Check sheet for the modelled part. Datum: model origin and axes. Units: mm. A direction names the side the tool comes from. Round coordinates to 2 decimals unless told otherwise and drop trailing zeros. Write each loop counter-clockwise with the first axis right and the second up, starting at its lowest first coordinate (ties: lowest second). Pieces come first, ordered by that corner, then holes.
Item 1: Depth check by flat-ended pin: pin 1 (5 mm diameter, centred on x = -133.5, z = -11.5, fed in from -Y); pin 2 (5 mm diameter, centred on x = 62.5, y = -26.5, fed in from -Z); pin 3 (4 mm diameter, centred on y = -3, z = -67, fed in from -X). Enter the tip coordinate at first touch or a pass-through.
Item 2: Material ranges on line 1 along Z through (x, y) = (-70, -9.5); line 2 along Y through (x, z) = (110, -3.5); line 3 along X through (y, z) = (-4, 32.5), recorded low to high.
Item 3: Section check D-D, the plane x = 111. Record the cut outline in (y, z).
Item 4: Section check A-A, the plane z = -79. Record the cut outline in (x, y).
Item 5: Set-up check for faces 1 (the flat face through (102.829, -17, -1)), 2 (the flat face through (-4, -15, -95)), 3 (the flat face through (-107.171, -17, -1)): record each of +Z, -Z, +X, -X, +Y, -Y from which the full face is reachable in a straight line by a thin tool's end or side.
Item 6: Section check C-C, the plane y = -17. Record the cut outline in (x, z), plus the area to 3 significant figures.
Item 7: Section check B-B, the plane x = -93.5. Record the cut outline in (y, z).
from build123d import *

# Parameters (mm, degrees)
F0_W     = 210
F0_H     = 190
F1_DEPTH = 40
F2_W     = 330
F2_H     = 310
F3_DEPTH = 30
F4_SIZE  = 10
F5_SIZE  = 5


with BuildPart() as f1:
    # F0 (on Front) → F1 (new body)
    with BuildSketch(Plane.XZ):
        with Locations((-2.170864, 0)):
            Rectangle(F0_W, F0_H)
    extrude(amount=F1_DEPTH)

    # F2 (on face) → F3 (join)
    with BuildSketch(Plane(origin=(0, 0, 0), x_dir=(-1, 0, 0), z_dir=(0, 1, 0))):
        with Locations((2.170864, 0)):
            Rectangle(F2_W, F2_H)
    extrude(amount=F3_DEPTH)

    # F4
    f4_edges = [f1.edges().sort_by_distance(p)[0] for p in [
        (-2.170864, -40, 95),
        (-2.170864, -40, -95),
    ]]
    chamfer(f4_edges, length=F4_SIZE)

    # F5
    f5_edges = [f1.edges().sort_by_distance(p)[0] for p in [
        (-107.170864, -40, 0),
        (102.829136, -40, 0),
    ]]
    chamfer(f5_edges, length=F5_SIZE)


solid = f1.part
Values found:
1. pin 1: stops at y = 0
1. pin 2: stops at z = -95
1. pin 3: stops at x = -107.17
2. line 1: z = -95 to 95
2. line 2: y = 0 to 30
2. line 3: x = -107.17 to 102.83
3. outline: (0, -155) - (30, -155) - (30, 155) - (0, 155) - close
4. outline: (-167.17, 0) - (-107.17, 0) - (-107.17, -35) - (-102.17, -40) - (97.83, -40) - (102.83, -35) - (102.83, 0) - (162.83, 0) - (162.83, 30) - (-167.17, 30) - close
5. face 1: +Z, -Z, +X, -Y
5. face 2: -Z, +X, -X, -Y
5. face 3: +Z, -Z, -X, -Y
6. outline: (-107.17, -95) - (102.83, -95) - (102.83, 95) - (-107.17, 95) - close
6. area: 39,900 mm2
7. outline: (-40, -85) - (-30, -95) - (0, -95) - (0, -155) - (30, -155) - (30, 155) - (0, 155) - (0, 95) - (-30, 95) - (-40, 85) - close
